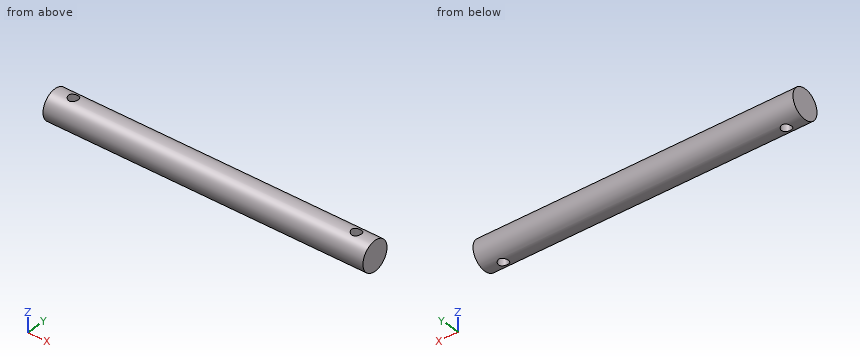
from build123d import *

# Parameters (mm, degrees)
SKETCH1_W               = 130
SKETCH1_H               = 6
CUT_EXTRUDE6_DEPTH      = 131.276628756
CUT_EXTRUDE6_DEPTH_BACK = 131.276628756
SKETCH2_R               = 2
CUT_EXTRUDE7_DEPTH      = 131.276628865
CUT_EXTRUDE7_DEPTH_BACK = 131.276628865
SKETCH2_7_R             = 2


with BuildPart() as part:
    # Sketch1 → Revolve1 (revolve)
    with BuildSketch(Plane.XY, mode=Mode.PRIVATE) as revolve1_sk:
        with Locations((65, 3)):
            Rectangle(SKETCH1_W, SKETCH1_H)
    revolve(revolve1_sk.sketch.rotate(Axis((0, 0, 0), (1, 0, 0)), 90), axis=Axis((0, 0, 0), (1, 0, 0)))

    # Sketch2 → Cut-Extrude6 (cut, two sides: drawn at the far end of the back side and taken through both)
    with BuildSketch(Plane.XY.offset(-CUT_EXTRUDE6_DEPTH_BACK)):
        with Locations((7.5, 0)):
            Circle(SKETCH2_R)
    extrude(amount=CUT_EXTRUDE6_DEPTH + CUT_EXTRUDE6_DEPTH_BACK, mode=Mode.SUBTRACT)

    # Sketch2_7 → Cut-Extrude7 (cut, two sides: drawn at the far end of the back side and taken through both)
    with BuildSketch(Plane.XY.offset(-CUT_EXTRUDE7_DEPTH_BACK)):
        with Locations((122.5, 0)):
            Circle(SKETCH2_7_R)
    extrude(amount=CUT_EXTRUDE7_DEPTH + CUT_EXTRUDE7_DEPTH_BACK, mode=Mode.SUBTRACT)


solid = part.part
Build history of the part. All positions in model axes, mm. Coordinates: 2 decimals unless noted, no trailing zeros. Order: outer loops, then holes, each group sorted by start corner. A loop starts at its lowest first (then second) coordinate and runs counter-clockwise, first axis right, second up. Notation, with made-up numbers: (-24.75, -17) - (-4.75, -17) arc R20 ccw to (-4.75, 3) - close; hole circle Ø9 at (2.5, 87.25). An arc over 180 degrees is marked (long way). Put each result on its own line as item: value.
1. Saw through at B-B (z = 0). Write the cut outline in (x, y).
Answer sheet:
outline: (0, -6) - (130, -6) - (130, 6) - (0, 6) - close; hole circle Ø4 at (7.5, 0); hole circle Ø4 at (122.5, 0)
2. Probe line 1 along X through (y, z) = (0, -0.75); line 2 along Y through (x, z) = (122.5, 0.25); line 3 along Y through (x, z) = (95.5, 0.5). List the from-to ranges inside material, lowest first. Write a range as [from, to].
Answer sheet:
line 1: x = [0, 5.5], [9.5, 120.5], [124.5, 130]
line 2: y = [-5.99, -2], [2, 5.99]
line 3: y = [-5.98, 5.98]
3. Saw through at C-C (x = 7.5). Write the cut outline in (y, z), and give its area (3 significant figures).
Answer sheet:
outline: (-2, -5.66) - (-2, 5.66) arc R6 ccw to start; (2, -5.66) arc R6 ccw to (2, 5.66) - close
area: 66.0 mm^2
4. Saw through at D-D (x = 41). Write the cut outline in (y, z).
Answer sheet:
outline: circle Ø12 at (0, 0)
5. Drop flat-ended pins along their axis: P1, Ø4, axis at y = 2.5, z = -0.5, coming from the -X side; P2, Ø3, axis at x = 89.5, z = -2.5, coming from the +Y side; P3, Ø1.5, axis at x = 47.5, z = 1, coming from the +Y side; P4, Ø1.5, axis at x = 89.5, z = -3, coming from the +Y side. Give the stop position or say it passes through.
Answer sheet:
P1: stops at x = 0
P2: stops at y = 5.92
P3: stops at y = 5.99
P4: stops at y = 5.56
6. Saw through at A-A (y = 0). Write the cut outline in (x, z).
Answer sheet:
outline: (0, -6) - (5.5, -6) - (5.5, 6) - (0, 6) - close; (9.5, -6) - (120.5, -6) - (120.5, 6) - (9.5, 6) - close; (124.5, -6) - (130, -6) - (130, 6) - (124.5, 6) - close
